Geometry: final body of the model. Coordinates: model frame, mm. Face numbers are marked on the shaded views. A direction names the side the tool comes from. Give positions to 0.01 mm unless a question says otherwise; leave off trailing zeros. Write each loop counter-clockwise with the first axis right and the second up, starting at its lowest first coordinate (ties: lowest second). Pieces come first, ordered by that corner, then holes.
Q1. Section C-C (y = 8.5). Return the cut outline in (x, z).
Q2. Pin query (flat end, axial travel): pin 1 Ø1.5 at (x, z) = (-12.5, 4.5) entering from -Y; pin 2 Ø1 at (y, z) = (-14, 0.5) entering from +X; pin 3 Ø5 at (x, y) = (-7.5, 10) entering from -Z; pin 4 Ø1 at (x, z) = (-9.5, 2.5) entering from +Y. Return the tip coordinate at first contact, or that it passes through.
Q3. Reachability of the marked faces 1 and 2 from +Z, -Z, +X, -X, +Y, -Y: full face, straight path, thin tool, end or side. Return the list, or none.
Q4. Section B-B (z = 3.5). State how many separate pieces and enclosed holes the cut face has, plus the area to 3 significant figures.
Q5. Section A-A (y = -15). Return the cut outline in (x, z), plus the area to 3 significant figures.
Q6. Mould query, pull axis X, two halves, no side actions, for the marked faces 3, 4 and 5. Classes: +X half, -X half, draft (parallel to the pull), parting line (faces both ways), or undercut.
Q7. Section D-D (y = 16). Return the cut outline in (x, z).
Q8. Line query: line 1 (Y direction, x = -7.5, z = 0.3); line 2 (Y direction, x = -5, z = 3.7); line 3 (X direction, y = -0.5, z = 3.55). Output: solid intervals per line, ascending.
from build123d import *

# Parameters (mm, degrees)
ESQUISSE1_R        = 19
ESQUISSE1_R_2      = 1.5
BOSS_EXTRU_2_DEPTH = 6


with BuildPart() as part:
    # Esquisse1 → Boss.-Extru.2 (new body)
    with BuildSketch(Plane.XY):
        Circle(ESQUISSE1_R)
        with Locations((-0.493805045, 13.991288596)):
            Circle(ESQUISSE1_R_2, mode=Mode.SUBTRACT)
        with Locations((12.363713879, -6.567996584)):
            Circle(ESQUISSE1_R_2, mode=Mode.SUBTRACT)
        with Locations((-11.869908833, -7.423292012)):
            Circle(ESQUISSE1_R_2, mode=Mode.SUBTRACT)
        with BuildLine():
            ThreePointArc((-0.379171731, 10.743310886), (0.922172629, 11.065966866), (1.982535482, 11.886475637))
            ThreePointArc((1.982535482, 11.886475637), (3.751818189, 12.953817976), (5.806908291, 12.738909534))
            ThreePointArc((5.806908291, 12.738909534), (9.198945104, 10.553644346), (11.826845368, 7.491710662))
            ThreePointArc((11.826845368, 7.491710662), (15.95449234, 6.343310094), (15.356979769, 2.100755188))
            ThreePointArc((15.356979769, 2.100755188), (15.472630931, 0.920701949), (15.497738971, -0.264739076))
            ThreePointArc((15.497738971, -0.264739076), (13.97233787, -1.738900356), (12.49817659, -0.213499254))
            ThreePointArc((12.49817659, -0.213499254), (12.485444687, 0.603051388), (12.419421545, 1.417028044))
            ThreePointArc((12.419421545, 1.417028044), (11.936947212, 1.58360629), (11.486503898, 1.823670062))
            ThreePointArc((11.486503898, 1.823670062), (10.947627516, 0.882480264), (10.748431867, -0.183609359))
            ThreePointArc((10.748431867, -0.183609359), (10.408589086, -2.687707806), (9.493566014, -5.043283091))
            ThreePointArc((9.493566014, -5.043283091), (9.122322109, -6.331608356), (9.302722122, -7.66016391))
            ThreePointArc((9.302722122, -7.66016391), (9.342426349, -9.72607885), (8.128765127, -11.398384864))
            ThreePointArc((8.128765127, -11.398384864), (4.540251554, -13.243342321), (0.574589068, -13.988203866))
            ThreePointArc((0.574589068, -13.988203866), (-2.483778485, -16.988650718), (-5.859182525, -14.3499122))
            ThreePointArc((-5.859182525, -14.3499122), (-6.938964188, -13.860042424), (-7.97814025, -13.289066113))
            ThreePointArc((-7.97814025, -13.289066113), (-8.492100818, -11.230949368), (-6.433984073, -10.7169888))
            ThreePointArc((-6.433984073, -10.7169888), (-5.720464522, -11.11423797), (-4.982528488, -11.464048581))
            ThreePointArc((-4.982528488, -11.464048581), (-4.597030329, -11.129502674), (-4.163907347, -10.859439207))
            ThreePointArc((-4.163907347, -10.859439207), (-4.709563431, -9.922163672), (-5.533226303, -9.216610368))
            ThreePointArc((-5.533226303, -9.216610368), (-7.53191778, -7.670248663), (-9.114394283, -5.700027795))
            ThreePointArc((-9.114394283, -5.700027795), (-10.044494737, -4.73435851), (-11.285257604, -4.226311727))
            ThreePointArc((-11.285257604, -4.226311727), (-13.094244538, -3.227739126), (-13.935673418, -1.34052467))
            ThreePointArc((-13.935673418, -1.34052467), (-13.739196658, 2.689697975), (-12.401434435, 6.496493204))
            ThreePointArc((-12.401434435, 6.496493204), (-13.470713855, 10.645340625), (-9.497797245, 12.249157012))
            ThreePointArc((-9.497797245, 12.249157012), (-8.533666743, 12.939340475), (-7.519598721, 13.553805188))
            ThreePointArc((-7.519598721, 13.553805188), (-5.480237052, 12.969849724), (-6.064192517, 10.930488055))
            ThreePointArc((-6.064192517, 10.930488055), (-6.764980165, 10.511186582), (-7.436893057, 10.047020536))
            ThreePointArc((-7.436893057, 10.047020536), (-7.339916883, 9.545896384), (-7.32259655, 9.035769145))
            ThreePointArc((-7.32259655, 9.035769145), (-6.238064085, 9.039683408), (-5.215205564, 9.400219727))
            ThreePointArc((-5.215205564, 9.400219727), (-2.876671305, 10.357956468), (-0.379171731, 10.743310886))
        make_face(mode=Mode.SUBTRACT)
    extrude(amount=BOSS_EXTRU_2_DEPTH)


solid = part.part
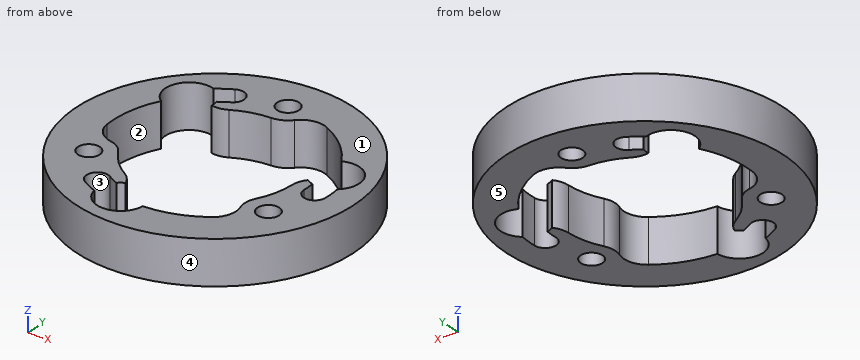
Computed:
1. outline: (-16.99, 0) - (-13.75, 0) - (-13.75, 6) - (-16.99, 6) - close; (11.12, 0) - (16.99, 0) - (16.99, 6) - (11.12, 6) - close
2. pin 1: stops at y = -14.93
2. pin 2: stops at x = 13.37
2. pin 3: stops at z = 0
2. pin 4: stops at y = 16.73
3. face 1: +Z, +X, -X, +Y, -Y
3. face 2: +Z, -Z
4. separate pieces: 1
4. enclosed holes: 4
4. area: 519 mm2
5. outline: (-11.66, 0) - (-5.66, 0) - (-5.66, 6) - (-11.66, 6) - close; (0.33, 0) - (11.66, 0) - (11.66, 6) - (0.33, 6) - close
5. area: 104 mm2
6. face 3: undercut
6. face 4: parting line
6. face 5: draft
7. outline: (-10.25, 0) - (10.25, 0) - (10.25, 6) - (-10.25, 6) - close
8. line 1: y = -17.46 to -13.56, -10.53 to -7.7, 13.56 to 17.46
8. line 2: y = -18.33 to -16.01, -11.46 to -9.62, 9.52 to 18.33
8. line 3: x = -18.99 to -13.99, 10.74 to 12.52, 15.48 to 18.99
